Autodesk Inventor part; units mm, degrees
ref_plane "YZ Plane" through (0, 0, 0) normal (1, 0, 0) x (0, 1, 0)
ref_plane "XZ Plane" through (0, 0, 0) normal (0, 1, 0) x (-1, 0, 0)
ref_plane "XY Plane" through (0, 0, 0) normal (0, 0, 1) x (1, 0, 0)
sketch "Sketch1" plane through (0, 0, 0) normal (0, 1, 0) x (-1, 0, 0)
  line L0 (0, 0) -> (35, 0)
  line L1 (35, 0) -> (35, -50)
  line L2 (35, -50) -> (0, -50)
  line L3 (0, -50) -> (0, 0)
  line L4 (0, 0) -> (0, -10)
  line L5 (0, -10) -> (0, -20)
  line L6 (0, -20) -> (0, -30)
  line L7 (0, -30) -> (0, -40)
  line L8 (35, 0) -> (35, -10)
  line L9 (35, -10) -> (35, -20)
  line L10 (35, -20) -> (35, -30)
  line L11 (35, -30) -> (35, -40)
  circle A0 centre (35, 0) radius 1.5
  circle A1 centre (35, -10) radius 1.5
  circle A2 centre (35, -20) radius 1.5
  circle A3 centre (35, -30) radius 1.5
  circle A4 centre (35, -40) radius 1.5
  circle A5 centre (35, -50) radius 1.5
  circle A6 centre (0, -50) radius 1.5
  circle A7 centre (0, -40) radius 1.5
  circle A8 centre (0, -30) radius 1.5
  circle A9 centre (0, -20) radius 1.5
  circle A10 centre (0, -10) radius 1.5
  circle A11 centre (0, 0) radius 1.5
  line L12 (35, -50) -> (38, -50)
  line L13 (38, -50) -> (38, -53)
  line L14 (38, -53) -> (35, -53)
  line L15 (35, -53) -> (35, -50)
  line L16 (0, 0) -> (-3, 0)
  line L17 (-3, 0) -> (-3, 3)
  line L18 (-3, 3) -> (0, 3)
  line L19 (0, 3) -> (0, 0)
  line L20 (-3, 3) -> (38, 3)
  line L21 (38, 3) -> (38, -53)
  line L22 (38, -53) -> (-3, -53)
  line L23 (-3, -53) -> (-3, 3)
  line L24 (35, 0) -> (0, 0)
  line L25 (0, 0) -> (0, -10)
  line L26 (0, -10) -> (35, -10)
  line L27 (35, -10) -> (35, 0)
  line L28 (35, -10) -> (0, -10)
  line L29 (0, -10) -> (0, -20)
  line L30 (0, -20) -> (35, -20)
  line L31 (35, -20) -> (35, -10)
  line L32 (35, -20) -> (0, -20)
  line L33 (0, -20) -> (0, -30)
  line L34 (0, -30) -> (35, -30)
  line L35 (35, -30) -> (35, -20)
  line L36 (35, -30) -> (0, -30)
  line L37 (0, -30) -> (0, -40)
  line L38 (0, -40) -> (35, -40)
  line L39 (35, -40) -> (35, -30)
  line L40 (35, 0) -> (32, 0)
  line L41 (32, 0) -> (32, -50)
  line L42 (32, -50) -> (35, -50)
  line L43 (35, -50) -> (35, 0)
  line L44 (0, 0) -> (3, 0)
  line L45 (3, 0) -> (3, -50)
  line L46 (3, -50) -> (0, -50)
  line L47 (0, -50) -> (0, 0)
  point P0 (32, 0)
  point P1 (32, -10)
  point P2 (3, -10)
  point P3 (3, -40)
  point P4 (32, -40)
  point P5 (3, -20)
  point P6 (32, -20)
  point P7 (32, -30)
  point P8 (3, -30)
  dimension "d0" = 35
  dimension "d1" = 50
  dimension "d2" = 10
  dimension "d3" = 10
  dimension "d4" = 10
  dimension "d5" = 10
  dimension "d6" = 10
  dimension "d7" = 10
  dimension "d8" = 10
  dimension "d9" = 10
  dimension "d10" = 3
  dimension "d11" = 3
  dimension "d12" = 3
  dimension "d13" = 3
  dimension "d14" = 3
  dimension "d15" = 3
  dimension "d16" = 3
  dimension "d17" = 3
  dimension "d18" = 3
  dimension "d19" = 3
  dimension "d20" = 3
  dimension "d21" = 3
  dimension "d22" = 3
  dimension "d23" = 3
  dimension "d24" = 3
  dimension "d25" = 3
  dimension "d26" = 3
  dimension "d27" = 3
extrude "Extrusion1" add sketch "Sketch1" along normal blind 3 contours A11 L19 L20 L21 L12 A5 L1 A4 A3 A2 A1 A0 L0 | L0 L45 L26 A10 L3 A11 | L3 A10 A9 A8 A7 A6 L2 A5 L15 L22 L23 L16 A11 | L16 L17 L18 L19 A11 | L0 A0 L1 A1 L26 L41 | L45 L30 A9 L3 A10 L26 | L26 L41 L30 L45 | L26 A1 L1 A2 L30 L41 | L45 L34 A8 L3 A9 L30 | L15 A5 L12 L13 L14 | L30 A2 L1 A3 L34 L41 | L45 L38 A7 L3 A8 L34 | L34 L41 L38 L45 | L34 A3 L1 A4 L38 L41 | L45 L2 A6 L3 A7 L38 | L2 L41 L38 A4 L1 A5
fillet "Fillet1" radius 3 16 edges at (3, 1.5, 3) (-38, 1.5, 3) (-38, 1.5, -53) (3, 1.5, -53) (-32, 1.5, -50) (-32, 1.5, -40) (-3, 1.5, -40) (-3, 1.5, -50) (-3, 1.5, -30) (-3, 1.5, -20) (-32, 1.5, -20) (-32, 1.5, -30) (-32, 1.5, -10) (-32, 1.5, 0) (-3, 1.5, 0) (-3, 1.5, -10)
properties part number "base_extender"
Model file for the job. Use its own axes, mm. A direction names the side the tool comes from. Round coordinates to 2 decimals unless told otherwise and drop trailing zeros. Order: outer loops, then holes, each group sorted by start corner. A loop starts at its lowest first (then second) coordinate and runs counter-clockwise, first axis right, second up. Notation, with made-up numbers: M 34.5,50.25 L 50.5,50.25 A18 cw 50.5,74.25 Z; hole C 61.25,-4.75 d8. An arc over 180 degrees is marked long. Use CSV: the item, a comma, the result in double quotes.
Item 1: Pull direction X, two halves, no side cores. Call faces 1 (the face through (-38, 1, -25)), 2 (the face through (-17, 1, -20)), 3 (the face through (-17, 1, 3)): released by +X, released by -X, zero draft, split by the parting line, or undercut.
Worked answers:
face 1,"released by -X"
face 2,"undercut"
face 3,"zero draft"
Item 2: Which spindle directions (+Z, -Z, +X, -X, +Y, -Y) get a long thin tool onto all of the face, cutting with end or side? Do faces 4 (the face through (2.14, 1.52, -52.1)), 5 (the face through (-17, 1, 0)). Say none if no direction does.
Worked answers:
face 4,"-Z, +X, +Y, -Y"
face 5,"+Y, -Y"
Item 3: Saw through at C-C (y = 1.95). State how many separate pieces and enclosed holes the cut face has, plus the area to 3 significant figures.
Worked answers:
separate pieces,"1"
enclosed holes,"15"
area,"1,360 mm²"
Item 4: Probe probe 1 along Z at (x, y) = (-23.5, 1.2); probe 2 along X at (y, z) = (2.3, -10.5); probe 3 along X at (y, z) = (0.2, -6.5). List the from-to ranges inside material, lowest first.
Worked answers:
probe 1,"-53 to -50, -40 to -30, -20 to -10, 0 to 3"
probe 2,"-38 to -36.41, -33.59 to -1.41, 1.41 to 3"
probe 3,"-38 to -32, -3 to 3"
Item 5: Pin check, flat tip, straight feed: pin 1 (2.5 mm diameter, centred on x = -35, z = -50, fed in from -Y). Stop position of the tip, or through.
Worked answers:
pin 1,"through"
Item 6: Saw through at A-A (z = -5). List the corners of the cut face in (x, y), plus the area to 3 significant figures.
Worked answers:
outline,"M -38,0 L -32,0 L -32,3 L -38,3 Z; M -3,0 L 3,0 L 3,3 L -3,3 Z"
area,"36.0 mm²"
Item 7: Saw through at B-B (x = -19). List the corners of the cut face in (y, z), plus the area to 3 significant figures.
Worked answers:
outline,"M 0,-53 L 3,-53 L 3,-50 L 0,-50 Z; M 0,-40 L 3,-40 L 3,-30 L 0,-30 Z; M 0,-20 L 3,-20 L 3,-10 L 0,-10 Z; M 0,0 L 3,0 L 3,3 L 0,3 Z"
area,"78.0 mm²"
